Geometry check sheet. Reference: the model listing, model coordinates, mm. Face numbers are marked on the shaded views. A direction names the side the tool comes from. Coordinates: 2 decimals unless noted, no trailing zeros. Order: outer loops, then holes, each group sorted by start corner. A loop starts at its lowest first (then second) coordinate and runs counter-clockwise, first axis right, second up. Notation, with made-up numbers: (44, 29.25) -> (50, 29.25) arc R22 ccw to (50, 60.25) -> close; hole circle Ø10 at (77.5, 89.25). An arc over 180 degrees is marked (long way). Answer in a Markdown table with one row per item. Add a question column.
```python
from build123d import *

# Parameters (mm, degrees)
SKETCH1_R           = 1.25
BOSS_EXTRUDE1_DEPTH = 10
CUT_EXTRUDE1_REACH  = 89.179
SKETCH2_R           = 3
SKETCH3_R           = 7.5
SKETCH3_R_2         = 3
BOSS_EXTRUDE2_DEPTH = 3


with BuildPart() as part:
    # Sketch1 → Boss-Extrude1 (new body)
    with BuildSketch(Plane.XY):
        with BuildLine():
            Line((0.25, -3.240370349), (0.25, -80.240370349))
            ThreePointArc((0.25, -80.240370349), (1.919491347, -84.270879002), (5.95, -85.940370349))
            Line((5.95, -85.940370349), (10.95, -85.940370349))
            Line((10.95, -85.940370349), (10.95, -82.940370349))
            Line((10.95, -82.940370349), (5.95, -82.940370349))
            ThreePointArc((5.95, -82.940370349), (4.040811691, -82.149558658), (3.25, -80.240370349))
            Line((3.25, -80.240370349), (3.25, 0))
            ThreePointArc((3.25, 0), (-2.384848004, 2.207940217), (0.25, -3.240370349))
        make_face()
        Circle(SKETCH1_R, mode=Mode.SUBTRACT)
    extrude(amount=BOSS_EXTRUDE1_DEPTH)

    # Sketch2 → Cut-Extrude1 (cut, up to next)
    with BuildSketch(Plane.ZY.offset(-0.25), mode=Mode.PRIVATE) as cut_extrude1_sk1:
        with Locations(Location((5, -30.5, 0), (0, 0, 270))):
            Circle(SKETCH2_R)
    cut_extrude1_tool1 = extrude(cut_extrude1_sk1.sketch, amount=-CUT_EXTRUDE1_REACH, mode=Mode.PRIVATE) & part.part
    add(cut_extrude1_tool1.solids().sort_by_distance((0.25, -30.5, 5))[0], mode=Mode.SUBTRACT)

    # Sketch3 → Boss-Extrude2 (add)
    with BuildSketch(Plane.ZY.offset(-0.25)):
        with Locations((5, -30.5)):
            Circle(SKETCH3_R)
        with Locations(Location((5, -30.5, 0), (0, 0, 270))):
            Circle(SKETCH3_R_2, mode=Mode.SUBTRACT)
    extrude(amount=-BOSS_EXTRUDE2_DEPTH)


solid = part.part
```
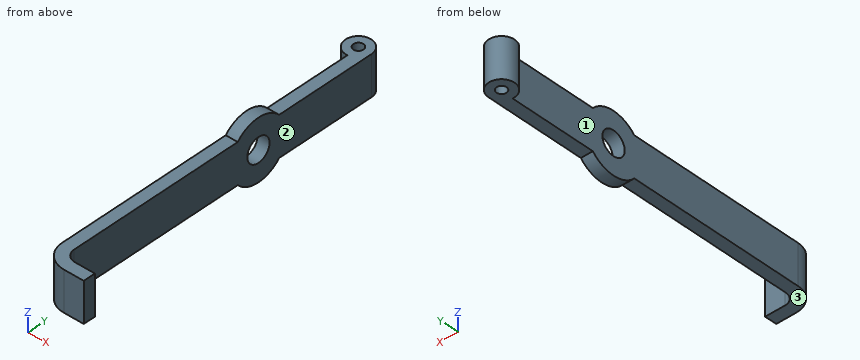
(1) Scan lines: line 1 along Z through (x, y) = (2.3, -30.5); line 2 along Y through (x, z) = (0, 3.5); line 3 along X through (y, z) = (-43, 3.5). Record each from-to range of solid material in increasing order.
(2) Cross-section at C-C (x = 9.5). Enter the section's corners in (y, z), plus the area to 3 significant figures.
(3) Go/stop test with flat-tipped pins: P1, Ø5, axis at x = 5, y = -31, coming from the +Z side; P2, Ø7, axis at x = -1.5, y = -5, coming from the +Z side; P3, Ø5, axis at x = -1, y = -5.5, coming from the -Z side; P4, Ø4.5, axis at y = -38.5, z = 6, coming from the -X side. Record where each tip stops, or that it passes through.
(4) Cross-section at B-B (y = -30.5). Enter the section's corners in (x, z).
(5) Cross-section at A-A (z = 5). Enter the section's corners in (x, y), plus the area to 3 significant figures.
(6) Access from +Z, -Z, +X, -X, +Y, -Y to the whole of each face (thin tool, end or side, straight path). Record for the marked faces 1, 2 and 3.
(7) Cross-section at D-D (y = -57). Enter the section's corners in (x, z).
Checks:
| question | item | result |
|---|---|---|
| 1 | line 1 | -2.5 to 2, 8 to 12.5 |
| 1 | line 2 | -3.25 to -1.25, 1.25 to 3.25 |
| 1 | line 3 | 0.25 to 3.25 |
| 2 | outline | (-85.94, 0) -> (-82.94, 0) -> (-82.94, 10) -> (-85.94, 10) -> close |
| 2 | area | 30.0 mm² |
| 3 | P1 | z = 12.5 |
| 3 | P2 | z = 10 |
| 3 | P3 | z = 0 |
| 3 | P4 | x = 0.25 |
| 4 | outline | (0.25, -2.5) -> (3.25, -2.5) -> (3.25, 2) -> (0.25, 2) -> close; (0.25, 8) -> (3.25, 8) -> (3.25, 12.5) -> (0.25, 12.5) -> close |
| 5 | outline | (0.25, -80.24) arc R5.7 ccw to (5.95, -85.94) -> (10.95, -85.94) -> (10.95, -82.94) -> (5.95, -82.94) arc R2.7 cw to (3.25, -80.24) -> (3.25, -33.5) -> (0.25, -33.5) -> close; (0.25, -27.5) -> (3.25, -27.5) -> (3.25, 0) arc R3.25 ccw (long way) to (0.25, -3.24) -> close; hole circle Ø2.5 at (0, 0) |
| 5 | area | 278 mm² |
| 6 | face 1 | +Z, -Z, -X, -Y |
| 6 | face 2 | +Z, -Z, +X, +Y |
| 6 | face 3 | -Z, +X, -X, -Y |
| 7 | outline | (0.25, 0) -> (3.25, 0) -> (3.25, 10) -> (0.25, 10) -> close |
